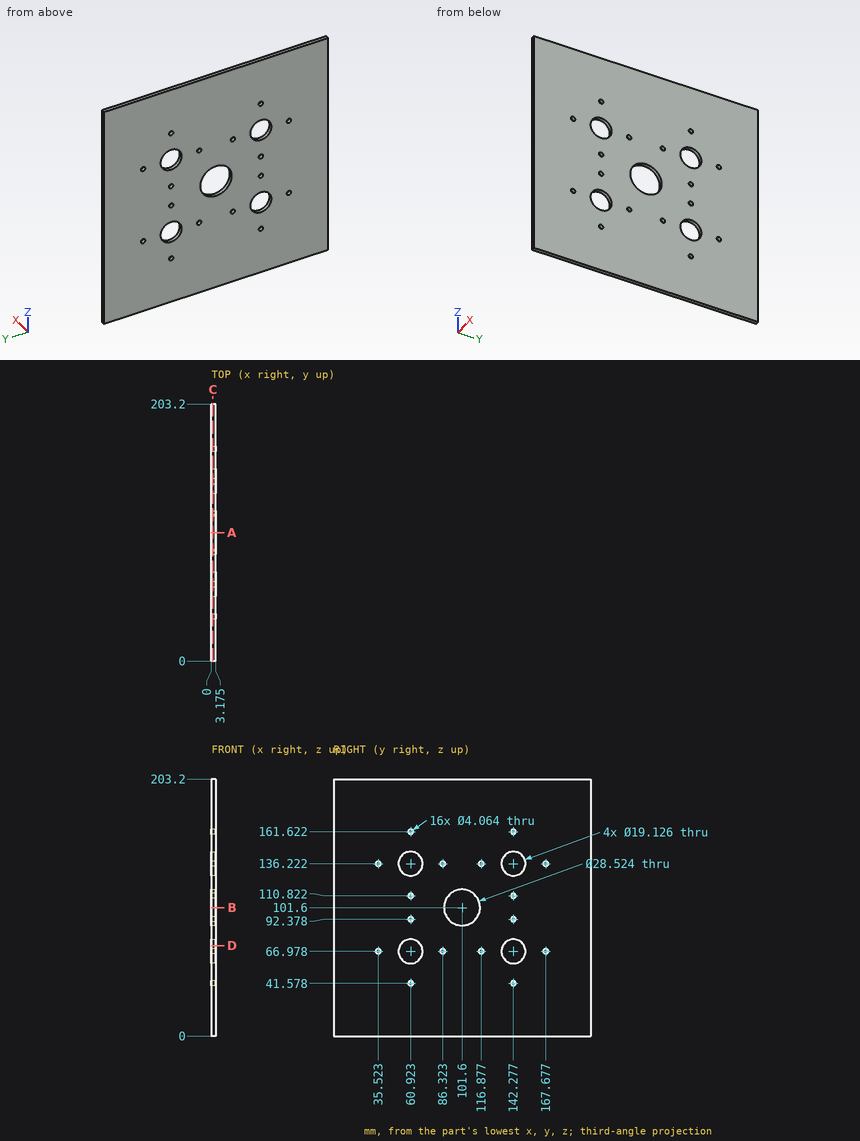
For this review, use the dimensioned drawing (mm, ordinates from the lowest corner) and the shaded views. Round coordinates to 2 decimals unless told otherwise and drop trailing zeros. Order: outer loops, then holes, each group sorted by start corner. A loop starts at its lowest first (then second) coordinate and runs counter-clockwise, first axis right, second up. Notation, with made-up numbers: M -17,25 L 11,25 A12 cw 11,43 Z; hole C 74,53.5 d6. An arc over 180 degrees is marked long. Use a Markdown table: item, result. Add a question column.
Item 1: Add section C-C, the plane x = 1.05. State how many separate pieces and enclosed holes the cut face has, then the cut area to 3 significant figures.
Item 2: To check wall thickness, follow line 1 along Y through (x, z) = (1.45, 162); line 2 along Z through (x, y) = (1.5, 117); line 3 along Y through (x, z) = (0.9, 93). State the ranges of each line that lie inside material, in increasing order.
Item 3: Add section D-D, the plane z = 71.5. Give the boundary of the cut face in (x, y) (1 decimal), then the cut area to 3 significant figures.
Item 4: Add section A-A, the plane y = 101.6. Give the boundary of the cut face in (x, z) (1 decimal).
Item 5: Insertion check: pin 1 (3.5 mm diameter, centred on y = 116.88, z = 66.98, fed in from -X). The pin has a flat end and moves straight along its axis. Give the tip position at first contact, or say it passes through.
Geometry results:
| question | item | result |
|---|---|---|
| 1 | separate pieces | 1 |
| 1 | enclosed holes | 21 |
| 1 | area | 39,300 mm² |
| 2 | line 1 | y = 0 to 58.93, 62.92 to 140.28, 144.27 to 203.2 |
| 2 | line 2 | z = 0 to 64.95, 69.01 to 134.19, 138.25 to 203.2 |
| 2 | line 3 | y = 0 to 58.99, 62.86 to 90.22, 112.98 to 140.34, 144.21 to 203.2 |
| 3 | outline | M 0,0 L 3.2,0 L 3.2,52.5 L 0,52.5 Z; M 0,69.3 L 3.2,69.3 L 3.2,133.9 L 0,133.9 Z; M 0,150.7 L 3.2,150.7 L 3.2,203.2 L 0,203.2 Z |
| 3 | area | 538 mm² |
| 4 | outline | M 0,0 L 3.2,0 L 3.2,87.3 L 0,87.3 Z; M 0,115.9 L 3.2,115.9 L 3.2,203.2 L 0,203.2 Z |
| 5 | pin 1 | passes through |
